Here's the drawing with two shaded views (mm, measured from the low corner). I have some questions. A direction names the side the tool comes from. Round coordinates to 2 decimals unless told otherwise and drop trailing zeros. Loops run counter-clockwise (first coordinate to the right, second up) from the corner with the lowest first, then second, coordinate; pieces in that order, holes last. Notation, with made-up numbers: M 11,-28.5 L 62,-28.5 A20 ccw 62,-15.5 Z; hole C 59.5,23 d11. An arc over 180 degrees is marked long. Answer as CSV lines item,"result".
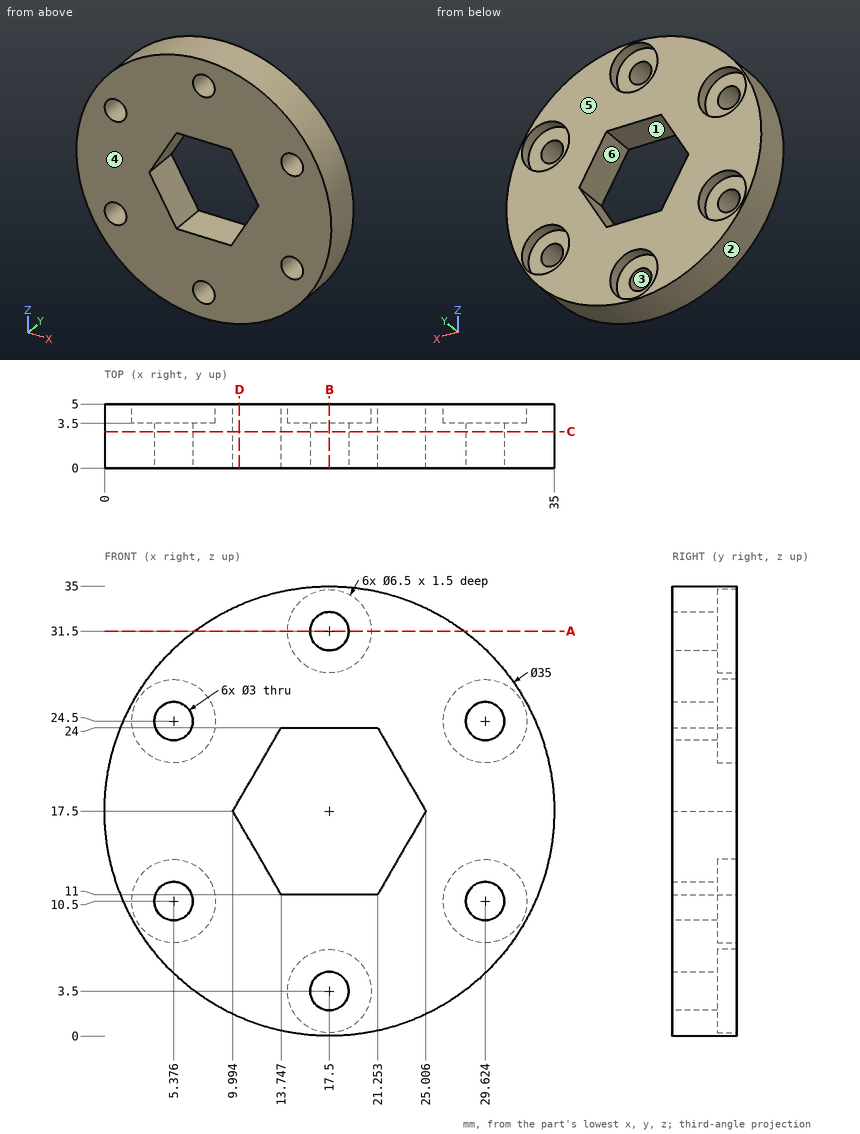
1. I want a section at C-C, the plane y = 2.85. Please give me the cut outline in (x, z) (1 decimal).
Evaluation:
outline,"C 17.5,17.5 d35; hole C 5.4,10.5 d3; hole C 5.4,24.5 d3; hole M 10,17.5 L 13.7,11 L 21.3,11 L 25,17.5 L 21.3,24 L 13.7,24 Z; hole C 17.5,3.5 d3; hole C 17.5,31.5 d3; hole C 29.6,10.5 d3; hole C 29.6,24.5 d3"
2. For P1, Ø3, axis at x = 28.5, z = 11, coming from the +Y side; P2, Ø2.5, axis at x = 5.38, z = 10.5, coming from the +Y side; P3, Ø2.5, axis at x = 16, y = 2, coming from the -Z side, each with a flat end and sliding along its axis, tell me the tip position at first contact or that it passes through.
Evaluation:
P1,"stops at y = 3.5"
P2,"passes through"
P3,"stops at z = 0"
3. I want a section at A-A, the plane z = 31.5. Please give me the cut outline in (x, y).
Evaluation:
outline,"M 7,0 L 16,0 L 16,3.5 L 14.25,3.5 L 14.25,5 L 7,5 Z; M 19,0 L 28,0 L 28,5 L 20.75,5 L 20.75,3.5 L 19,3.5 Z"
4. I want a section at B-B, the plane x = 17.5. Please give me the cut outline in (y, z).
Evaluation:
outline,"M 0,0 L 5,0 L 5,0.25 L 3.5,0.25 L 3.5,2 L 0,2 Z; M 0,5 L 3.5,5 L 3.5,6.75 L 5,6.75 L 5,11 L 0,11 Z; M 0,24 L 5,24 L 5,28.25 L 3.5,28.25 L 3.5,30 L 0,30 Z; M 0,33 L 3.5,33 L 3.5,34.75 L 5,34.75 L 5,35 L 0,35 Z"
5. Which directions (+Z, -Z, +X, -X, +Y, -Y) give clear straight access to the entire face, cutting with the end or side of a thin tool? Please do the marked faces 5 and 6.
Evaluation:
face 5,"+Z, -Z, +X, -X, +Y"
face 6,"+Y, -Y"
6. We'd pull the mould along X, two halves only. Please class the marked faces 1, 2, 3 and 4: pulls with the +X half, pulls with the -X half, needs draft (parallel to the pull), parting line crosses it, or undercut.
Evaluation:
face 1,"undercut"
face 2,"parting line crosses it"
face 3,"undercut"
face 4,"needs draft"
7. I want a section at D-D, the plane x = 10.5. Please give me the cut outline in (y, z) (1 decimal).
Evaluation:
outline,"M 0,1.5 L 5,1.5 L 5,16.6 L 0,16.6 Z; M 0,18.4 L 5,18.4 L 5,33.5 L 0,33.5 Z"
8. If I drill on line 1 (X direction, y = 1.35, z = 24.5) (1 decimal); line 2 (X direction, y = 0.55, z = 25.5) (1 decimal); line 3 (Z direction, x = 5.5, y = 1.7) (1 decimal), over which ranges is the centre line in solid material (lowest first)? Write a range as [from, to].
Evaluation:
line 1,"x = [1.5, 3.9], [6.9, 28.1], [31.1, 33.5]"
line 2,"x = [1.9, 4.3], [6.5, 28.5], [30.7, 33.1]"
line 3,"z = [4.8, 9], [12, 23], [26, 30.2]"
